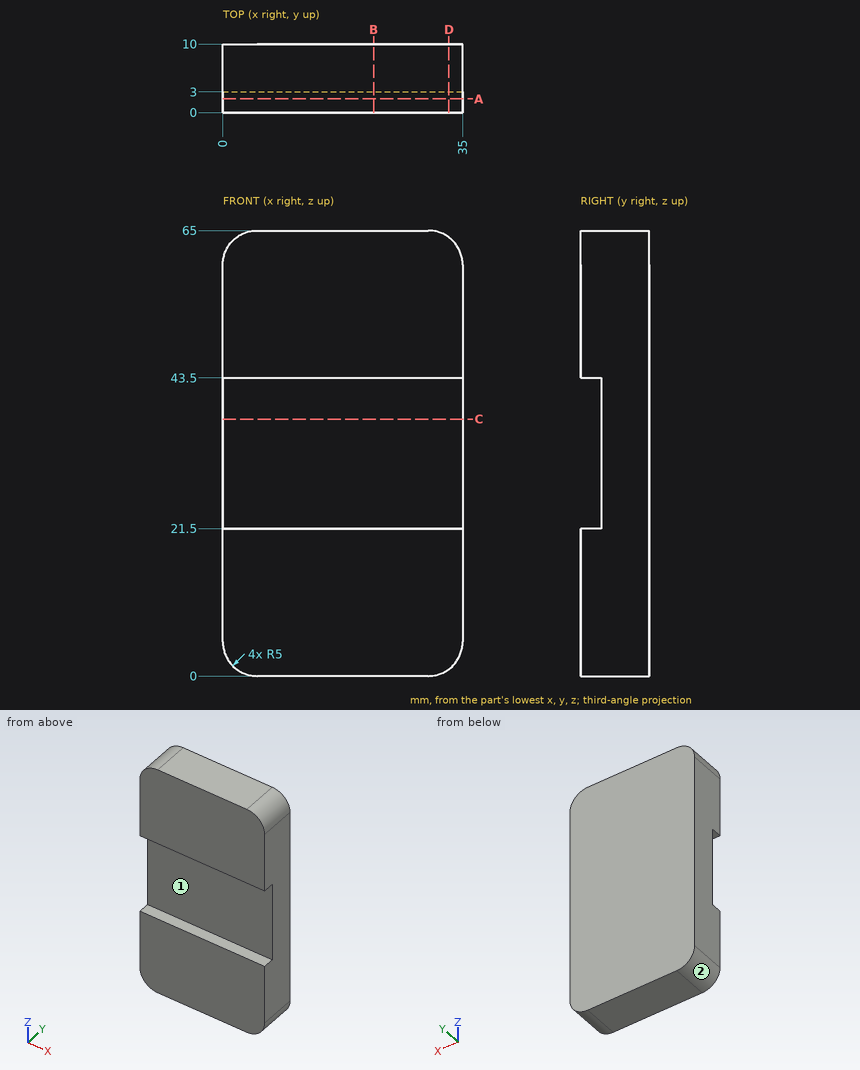
Study the drawing (mm; zero at the part's minimum x, y, z) and answer. A direction names the side the tool comes from. Round coordinates to 2 decimals unless told otherwise and drop trailing zeros. Order: outer loops, then holes, each group sorted by start corner. A loop starts at its lowest first (then second) coordinate and runs counter-clockwise, first axis right, second up. Notation, with made-up numbers: (37, 37) - (46, 37) arc R31 ccw to (46, 69) - close; hole circle Ø5 at (-17.5, 5.5). An arc over 180 degrees is marked (long way). Use one line per item in the form item = value. Start each with the question number.
(1) The part is cut by section D-D (x = 33). Give the vertices of the cut face in (y, z).
(2) The part is cut by section B-B (x = 22). Give the vertices of the cut face in (y, z).
(3) Find the intervals of material crossed by line 1 along Z through (x, y) = (10.5, 1.25); line 2 along Y through (x, z) = (13, 24); line 3 along Z through (x, y) = (3.5, 8.5), in increasing order. Write a range as from..to.
(4) For the marked faces 1 and 2, determine the directions among +Z, -Z, +X, -X, +Y, -Y from which every point of the face is accessible in a straight line to the end or side of a thin tool.
(5) The part is cut by section A-A (y = 2). Give the vertices of the cut face in (x, z).
(6) The part is cut by section C-C (z = 37.5). Give the vertices of the cut face in (x, y).
Checked values:
q1.outline = (0, 1) - (10, 1) - (10, 64) - (0, 64) - (0, 43.5) - (3, 43.5) - (3, 21.5) - (0, 21.5) - close
q2.outline = (0, 0) - (10, 0) - (10, 65) - (0, 65) - (0, 43.5) - (3, 43.5) - (3, 21.5) - (0, 21.5) - close
q3.line_1 = 0..21.5, 43.5..65
q3.line_2 = 3..10
q3.line_3 = 0.23..64.77
q4.face_1 = +X, -X, -Y
q4.face_2 = -Z, -X, +Y, -Y
q5.outline = (0, 5) arc R5 ccw to (5, 0) - (30, 0) arc R5 ccw to (35, 5) - (35, 21.5) - (0, 21.5) - close; (0, 43.5) - (35, 43.5) - (35, 60) arc R5 ccw to (30, 65) - (5, 65) arc R5 ccw to (0, 60) - close
q6.outline = (0, 3) - (35, 3) - (35, 10) - (0, 10) - close
